from build123d import *

# Parameters (mm, degrees)
F0_R     = 40
F0_R_2   = 2.5
F1_DEPTH = 25


with BuildPart() as f1:
    # F0 (on Front) → F1 (new body)
    with BuildSketch(Plane.XZ):
        Circle(F0_R)
        with BuildLine():
            ThreePointArc((-5, -30.594117), (-21.92031, -21.92031), (-30.594117, -5))
            Line((-30.594117, -5), (-5.59017, -5))
            ThreePointArc((-5.59017, -5), (-5.303301, -5.303301), (-5, -5.59017))
            Line((-5, -5.59017), (-5, -30.594117))
        make_face(mode=Mode.SUBTRACT)
        with BuildLine():
            Line((5, -30.594117), (5, -5.59017))
            ThreePointArc((5, -5.59017), (5.303301, -5.303301), (5.59017, -5))
            Line((5.59017, -5), (30.594117, -5))
            ThreePointArc((30.594117, -5), (21.92031, -21.92031), (5, -30.594117))
        make_face(mode=Mode.SUBTRACT)
        with BuildLine():
            Line((-5, 30.594117), (-5, 5.59017))
            ThreePointArc((-5, 5.59017), (-5.303301, 5.303301), (-5.59017, 5))
            Line((-5.59017, 5), (-30.594117, 5))
            ThreePointArc((-30.594117, 5), (-21.92031, 21.92031), (-5, 30.594117))
        make_face(mode=Mode.SUBTRACT)
        Circle(F0_R_2, mode=Mode.SUBTRACT)
        with BuildLine():
            ThreePointArc((5.59017, 5), (5.303301, 5.303301), (5, 5.59017))
            Line((5, 5.59017), (5, 30.594117))
            ThreePointArc((5, 30.594117), (21.92031, 21.92031), (30.594117, 5))
            Line((30.594117, 5), (5.59017, 5))
        make_face(mode=Mode.SUBTRACT)
    extrude(amount=F1_DEPTH)


solid = f1.part
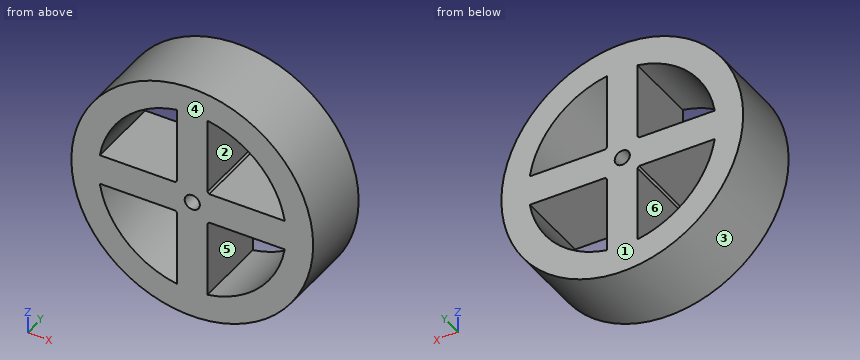
Build history of the part. All positions in model axes, mm. Face numbers are marked on the shaded views. A direction names the side the tool comes from. Coordinates: 2 decimals unless noted, no trailing zeros. Write each loop counter-clockwise with the first axis right and the second up, starting at its lowest first coordinate (ties: lowest second). Pieces come first, ordered by that corner, then holes.
(1) Cut at B-B on x = 0. List the corners of the cut face in (y, z).
(2) Mould opens along X. For the marked faces 3, 4, 5 and 6 say: pulls with the +X half, pulls with the -X half, needs draft (parallel to the pull), parting line crosses it, or undercut.
(3) Cut at D-D on x = 11. List the corners of the cut face in (y, z), and give its area (3 significant figures).
(4) Drill centre lines: line 1 (Z direction, x = 0, y = -5.5); line 2 (Z direction, x = -6.5, y = -15.5); line 3 (Z direction, x = -7, y = -14.5). Where is each one in solid material? Low to high.
(5) Cut at C-C on y = -8.5. List the corners of the cut face in (x, z).
(6) Pin check, flat tips, straight feed: pin 1 Ø8 at (y, z) = (-9, -31) entering from +X; pin 2 Ø7.5 at (y, z) = (-16.5, -18.5) entering from -X; pin 3 Ø7.5 at (x, y) = (21, -12.5) entering from +Z. Stop position of each tip, or through.
(7) Cut at A-A on z = 0. List the corners of the cut face in (x, y).
(8) 3-axis set-ups, long thin cutter, end or side, ignore diameter. For the marked faces 1 and 2: which of +Z, -Z, +X, -X, +Y, -Y reach the whole face in a straight line?
Working result:
1. outline: (-25, -40) - (0, -40) - (0, -2.5) - (-25, -2.5) - close; (-25, 2.5) - (0, 2.5) - (0, 40) - (-25, 40) - close
2. face 3: parting line crosses it
2. face 4: needs draft
2. face 5: undercut
2. face 6: undercut
3. outline: (-25, -38.46) - (0, -38.46) - (0, -28.98) - (-25, -28.98) - close; (-25, -5) - (0, -5) - (0, 5) - (-25, 5) - close; (-25, 28.98) - (0, 28.98) - (0, 38.46) - (-25, 38.46) - close
3. area: 724 mm2
4. line 1: z = -40 to -2.5, 2.5 to 40
4. line 2: z = -39.47 to -30.31, -5 to 5, 30.31 to 39.47
4. line 3: z = -39.38 to -30.2, -5 to 5, 30.2 to 39.38
5. outline: circle Ø80 at (0, 0); hole (-30.59, -5) arc R31 ccw to (-5, -30.59) - (-5, -5.59) arc R7.5 cw to (-5.59, -5) - close; hole (-30.59, 5) - (-5.59, 5) arc R7.5 cw to (-5, 5.59) - (-5, 30.59) arc R31 ccw to start; hole circle Ø5 at (0, 0); hole (5, -30.59) arc R31 ccw to (30.59, -5) - (5.59, -5) arc R7.5 cw to (5, -5.59) - close; hole (5, 5.59) arc R7.5 cw to (5.59, 5) - (30.59, 5) arc R31 ccw to (5, 30.59) - close
6. pin 1: stops at x = 29.51
6. pin 2: stops at x = -37.18
6. pin 3: stops at z = 36.09
7. outline: (-40, -25) - (-2.5, -25) - (-2.5, 0) - (-40, 0) - close; (2.5, -25) - (40, -25) - (40, 0) - (2.5, 0) - close
8. face 1: +Z, -Z, +X, -X, +Y
8. face 2: +Y, -Y
